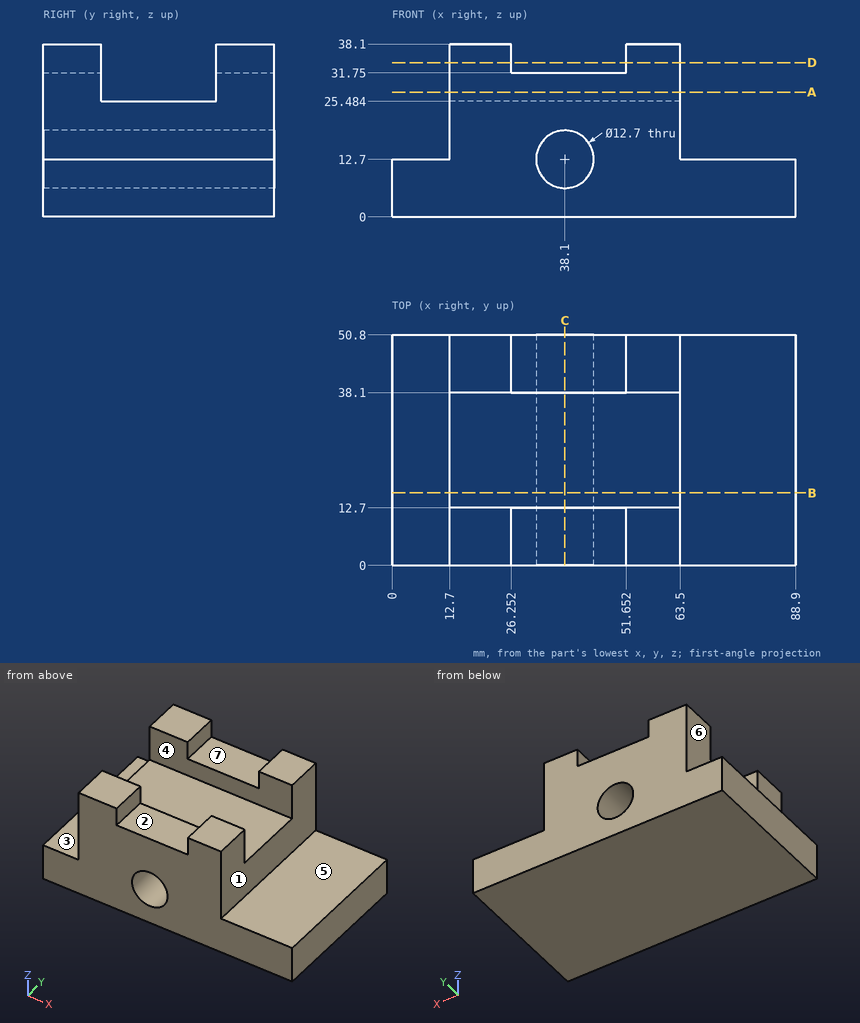
Study the drawing (mm; zero at the part's minimum x, y, z) and answer. A direction names the side the tool comes from. Round coordinates to 2 decimals unless told otherwise and drop trailing zeros. Loops run counter-clockwise (first coordinate to the right, second up) from the corner with the lowest first, then second, coordinate; pieces in that order, holes last.
Q1. Section D-D, the plane z = 34 is taken. Determine the outline of the cut face in (x, y), then the cut area to 3 significant figures.
Q2. Section C-C, the plane x = 38.1 is taken. Determine the outline of the cut face in (y, z).
Q3. Which of the six approach directions +Z, -Z, +X, -X, +Y, -Y give full straight-line access (tool end or side, diameter ignored) to the marked faces 1, 2, 3 and 4?
Q4. Section A-A, the plane z = 27.5 is taken. Determine the outline of the cut face in (x, y), then the cut area to 3 significant figures.
Q5. For a pull along X with two mould halves and no side action, classify the marked faces 5, 6 and 7 as released by +X, released by -X, zero draft, split by the parting line, or undercut.
Q6. Given pin 1 Ø4 at (y, z) = (34.5, 15.5) entering from +X; pin 2 Ø3 at (y, z) = (43.5, 36.5) entering from -X; pin 3 Ø6.5 at (x, y) = (32.5, 44.5) entering from +Z; pin 4 Ø14 at (x, z) = (37.5, 33.5) entering from +Y, each flat-ended and moving along its own axis, determine where each tip first touches the part or whether it passes through.
Q7. Section B-B, the plane y = 16 is taken. Determine the outline of the cut face in (x, z), then the cut area to 3 significant figures.
Q8. Find the intervals of material crossed by line 1 (X direction, y = 46, z = 36); line 2 (Y direction, x = 20.5, z = 31.5); line 3 (Z direction, x = 38, y = 18), in increasing order.
Completed:
1. outline: (12.7, 0) - (26.25, 0) - (26.25, 12.7) - (12.7, 12.7) - close; (12.7, 38.1) - (26.25, 38.1) - (26.25, 50.8) - (12.7, 50.8) - close; (51.65, 0) - (63.5, 0) - (63.5, 12.7) - (51.65, 12.7) - close; (51.65, 38.1) - (63.5, 38.1) - (63.5, 50.8) - (51.65, 50.8) - close
1. area: 645 mm2
2. outline: (0, 0) - (50.8, 0) - (50.8, 6.35) - (0, 6.35) - close; (0, 19.05) - (50.8, 19.05) - (50.8, 31.75) - (38.1, 31.75) - (38.1, 25.48) - (12.7, 25.48) - (12.7, 31.75) - (0, 31.75) - close
3. face 1: +Z, +X, +Y, -Y
3. face 2: +Z, +Y, -Y
3. face 3: +Z, -X, +Y, -Y
3. face 4: +Z, +X, -X
4. outline: (12.7, 0) - (63.5, 0) - (63.5, 12.7) - (12.7, 12.7) - close; (12.7, 38.1) - (63.5, 38.1) - (63.5, 50.8) - (12.7, 50.8) - close
4. area: 1,290 mm2
5. face 5: zero draft
5. face 6: released by -X
5. face 7: undercut
6. pin 1: stops at x = 63.5
6. pin 2: stops at x = 12.7
6. pin 3: stops at z = 31.75
6. pin 4: stops at y = 50.8
7. outline: (0, 0) - (88.9, 0) - (88.9, 12.7) - (63.5, 12.7) - (63.5, 25.48) - (12.7, 25.48) - (12.7, 12.7) - (0, 12.7) - close; hole circle Ø12.7 at (38.1, 12.7)
7. area: 1,650 mm2
8. line 1: x = 12.7 to 26.25, 51.65 to 63.5
8. line 2: y = 0 to 12.7, 38.1 to 50.8
8. line 3: z = 0 to 6.35, 19.05 to 25.48
